The model under review builds one solid part; all positions refer to its coordinate system, in mm. A direction names the side the tool comes from. Give positions to 0.01 mm unless a question says otherwise; leave off trailing zeros. Loops run counter-clockwise (first coordinate to the right, second up) from the corner with the lowest first, then second, coordinate; pieces in that order, holes last. Notation, with made-up numbers: M -21.75,26 L 11.25,26 A14 cw 11.25,50 Z; hole C -11.5,71.25 d5. An arc over 180 degrees is marked long. Put each result on its own line as item: value. Start each with the question number.
```python
from build123d import *

# Parameters (mm, degrees)
SKETCH1_R           = 5
BOSS_EXTRUDE1_DEPTH = 1.48
SKETCH2_R           = 4
BOSS_EXTRUDE2_DEPTH = 5.6
SKETCH3_R           = 1.6
CUT_EXTRUDE1_DEPTH  = 8.08
SKETCH4_R           = 3
CUT_EXTRUDE2_DEPTH  = 2


with BuildPart() as part:
    # Sketch1 → Boss-Extrude1 (new body)
    with BuildSketch(Plane(origin=(0, 0, 0), x_dir=(1, 0, 0), z_dir=(0, 1, 0))):
        Circle(SKETCH1_R)
    extrude(amount=BOSS_EXTRUDE1_DEPTH)

    # Sketch2 → Boss-Extrude2 (add)
    with BuildSketch(Plane(origin=(0, 1.48, 0), x_dir=(1, 0, 0), z_dir=(0, 1, 0))):
        Circle(SKETCH2_R)
    extrude(amount=BOSS_EXTRUDE2_DEPTH)

    # Sketch3 → Cut-Extrude1 (cut, through all)
    with BuildSketch(Plane.XZ):
        Circle(SKETCH3_R)
    extrude(amount=-CUT_EXTRUDE1_DEPTH, mode=Mode.SUBTRACT)

    # Sketch4 → Cut-Extrude2 (cut)
    with BuildSketch(Plane.XZ):
        Circle(SKETCH4_R)
    extrude(amount=-CUT_EXTRUDE2_DEPTH, mode=Mode.SUBTRACT)


solid = part.part
```
Item 1: Consider section A-A, the plane x = 0. Write out the cut boundary in (y, z), plus the area to 3 significant figures.
Item 2: Consider section D-D, the plane y = 6.5. Write out the cut boundary in (x, z), plus the area to 3 significant figures.
Item 3: Consider section C-C, the plane z = 2.25. Write out the cut boundary in (x, y), plus the area to 3 significant figures.
Item 4: To check wall thickness, follow L1, parallel to Z at x = 0, y = 6; L2, parallel to Z at x = -0.75, y = 1; L3, parallel to X at y = 4, z = -0.25. State the ranges of each line that lie inside material, in increasing order. Write a range as [from, to].
Item 5: Consider section B-B, the plane z = 0.25. Write out the cut boundary in (x, y).
Item 6: Draft analysis for pull direction X (two halves, no side actions). For faces 1 (the cylindrical face through (-3, 1, 0)), 2 (the cylindrical face through (-0.867, 4.241, 3.905)), 3 (the flat face through (2, 7.08, 0)), state which applies: +X half, -X half, draft (parallel to the pull), parting line (faces both ways), or undercut.
Item 7: Tool access review of faces 4 (the cylindrical face through (-1.08, 0.73, 4.88)), 5 (the flat face through (1.3, 2, -1.3)): name each direction out of +Z, -Z, +X, -X, +Y, -Y from which nothing blocks a thin tool from reaching the whole face with its end or side.
Item 8: Clearance check with flat-ended pins moving along their axes: pin 1 Ø3.5 at (x, z) = (0, 0) entering from -Y; pin 2 Ø1.5 at (y, z) = (4.5, -3.5) entering from -X; pin 3 Ø2.5 at (x, z) = (0, 0) entering from +Y; pin 4 Ø1 at (x, y) = (-2.5, 6) entering from +Z. State where each tip first meets the part, or that it passes through.
Report:
1. outline: M 0,-5 L 1.48,-5 L 1.48,-4 L 7.08,-4 L 7.08,-1.6 L 2,-1.6 L 2,-3 L 0,-3 Z; M 0,3 L 2,3 L 2,1.6 L 7.08,1.6 L 7.08,4 L 1.48,4 L 1.48,5 L 0,5 Z
1. area: 31.3 mm²
2. outline: C 0,0 d8; hole C 0,0 d3.2
2. area: 42.2 mm²
3. outline: M -4.47,0 L -1.98,0 L -1.98,2 L 1.98,2 L 1.98,0 L 4.47,0 L 4.47,1.48 L 3.31,1.48 L 3.31,7.08 L -3.31,7.08 L -3.31,1.48 L -4.47,1.48 Z
3. area: 42.3 mm²
4. L1: [-4, -1.6], [1.6, 4]
4. L2: [-4.94, -2.9], [2.9, 4.94]
4. L3: [-3.99, -1.58], [1.58, 3.99]
5. outline: M -4.99,0 L -2.99,0 L -2.99,2 L -1.58,2 L -1.58,7.08 L -3.99,7.08 L -3.99,1.48 L -4.99,1.48 Z; M 1.58,2 L 2.99,2 L 2.99,0 L 4.99,0 L 4.99,1.48 L 3.99,1.48 L 3.99,7.08 L 1.58,7.08 Z
6. face 1: undercut
6. face 2: parting line
6. face 3: draft
7. face 4: +Y, -Y
7. face 5: -Y
8. pin 1: y = 2
8. pin 2: x = -2.9
8. pin 3: through
8. pin 4: z = 3.46
